Source: three-view drawing plus pictorial views. Frame: mm from the lowest corner of the part. Give positions to 0.01 mm unless a question says otherwise; leave off trailing zeros. Order: outer loops, then holes, each group sorted by start corner. A loop starts at its lowest first (then second) coordinate and runs counter-clockwise, first axis right, second up. Notation, with made-up numbers: (25, -12.75) -> (57, -12.75) arc R27 cw to (57, 17.25) -> close; hole circle Ø2 at (47, -13). An arc over 180 degrees is marked (long way). Answer in a Markdown table with one row per item. Add a question column.
Q1. Line query: line 1 along Y through (x, z) = (12, 142.5); line 2 along Z through (x, y) = (42, 0.5); line 3 along X through (y, z) = (0.5, 19.5). Output: solid intervals per line, ascending. Write a range as from..to.
Q2. Contact query for flat-ended pins moving along their axis: P1, Ø4, axis at x = 43.5, y = 3.5, coming from the +Z side; P2, Ø1.5, axis at x = 86, y = 2.5, coming from the -Z side; P3, Ø5, axis at x = 78, z = 48.5, coming from the -Y side; P4, Ø1.5, axis at y = 2, z = 22.5, coming from the +X side. Output: stop coordinate, or through.
Q3. Cut plane B-B on x = 94. Return the cut outline in (y, z), and give its area (3 significant figures).
Q4. Cut plane D-D on x = 55.5. Return the cut outline in (y, z), and give its area (3 significant figures).
Q5. Cut plane C-C on y = 2. Return the cut outline in (x, z), and give its area (3 significant figures).
Q6. Cut plane A-A on z = 20. Return the cut outline in (x, y).
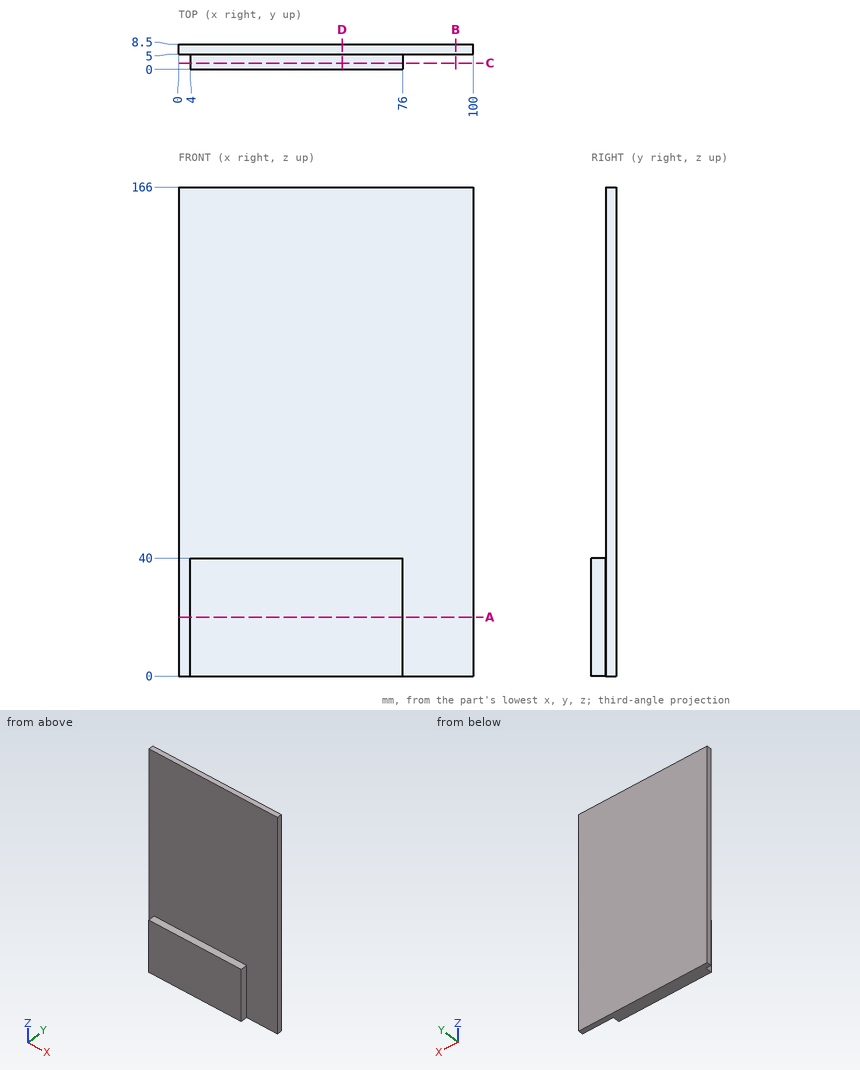
Completed:
| question | item | result |
|---|---|---|
| 1 | line 1 | y = 5..8.5 |
| 1 | line 2 | z = 0..40 |
| 1 | line 3 | x = 4..76 |
| 2 | P1 | stops at z = 166 |
| 2 | P2 | passes through |
| 2 | P3 | stops at y = 5 |
| 2 | P4 | stops at x = 76 |
| 3 | outline | (5, 0) -> (8.5, 0) -> (8.5, 166) -> (5, 166) -> close |
| 3 | area | 581 mm² |
| 4 | outline | (0, 0) -> (8.5, 0) -> (8.5, 166) -> (5, 166) -> (5, 40) -> (0, 40) -> close |
| 4 | area | 781 mm² |
| 5 | outline | (4, 0) -> (76, 0) -> (76, 40) -> (4, 40) -> close |
| 5 | area | 2,880 mm² |
| 6 | outline | (0, 5) -> (4, 5) -> (4, 0) -> (76, 0) -> (76, 5) -> (100, 5) -> (100, 8.5) -> (0, 8.5) -> close |
